from build123d import *

# Parameters (mm, degrees)
F0_W     = 200
F0_H     = 140
F1_DEPTH = 3
F2_R     = 10
F3_W     = 25
F3_H     = 50
F4_DEPTH = 20
F5_R     = 5
F6_DEPTH = 87.527208


with BuildPart() as f1:
    # F0 (on Front) → F1 (new body)
    with BuildSketch(Plane.XZ):
        with Locations((16.716758, -6.526925)):
            Rectangle(F0_W, F0_H)
    extrude(amount=F1_DEPTH)

    # F2
    f2_edges = [f1.edges().sort_by_distance(p)[0] for p in [
        (-83.283242, -1.5, -76.526925),
        (116.716758, -1.5, 63.473075),
        (116.716758, -1.5, -76.526925),
        (-83.283242, -1.5, 63.473075),
    ]]
    fillet(f2_edges, radius=F2_R)

    # F3 (on Front) → F4 (join)
    with BuildSketch(Plane.XZ):
        with Locations((129.216758, -6.526925)):
            Rectangle(F3_W, F3_H)
    extrude(amount=F4_DEPTH)

    # F5 (on face) → F6 (cut)
    with BuildSketch(Plane.XY.offset(18.473075)):
        with Locations((131.716758, -10)):
            Circle(F5_R)
    extrude(amount=-F6_DEPTH, mode=Mode.SUBTRACT)


solid = f1.part
Check sheet for the modelled part. Datum: model origin and axes. Units: mm. A direction names the side the tool comes from. Round coordinates to 2 decimals unless told otherwise and drop trailing zeros. Loops run counter-clockwise (first coordinate to the right, second up) from the corner with the lowest first, then second, coordinate; pieces in that order, holes last. Notation, with made-up numbers: M -28,25 L 9,25 A20 cw 9,45 Z; hole C -25,55 d7. An arc over 180 degrees is marked long. One line per item, written item: value.
(1) Depth check by flat-ended pin: pin 1 Ø2 at (x, z) = (112.5, 10) entering from -Y; pin 2 Ø5 at (y, z) = (-9, 4) entering from -X; pin 3 Ø0.9 at (y, z) = (-2, 27.5) entering from +X. Enter the tip coordinate at first touch or a pass-through.
Computed values:
pin 1: stops at y = -3
pin 2: stops at x = 116.72
pin 3: stops at x = 116.72
(2) Sectioned sample at D-D, the plane z = -64. Record the cut outline in (x, y), then the cut area to 3 significant figures.
Computed values:
outline: M -83.28,-3 L 116.72,-3 L 116.72,0 L -83.28,0 Z
area: 600 mm^2
(3) Sectioned sample at C-C, the plane x = 119. Record the cut outline in (y, z), then the cut area to 3 significant figures.
Computed values:
outline: M -20,-31.53 L 0,-31.53 L 0,18.47 L -20,18.47 Z
area: 1,000 mm^2
(4) Release check for a two-part mould opening along Y. For faces 1 (the face through (126, -10, -31.527)), 2 (the face through (28, 0, -6)), 3 (the face through (136.486, -8.498, -6.177)) record: +Y half, -Y half, draft (parallel to the pull), parting line (faces both ways), or undercut.
Computed values:
face 1: draft
face 2: +Y half
face 3: undercut
(5) Sectioned sample at B-B, the plane z = 6. Record the cut outline in (x, y).
Computed values:
outline: M -83.28,-3 L 116.72,-3 L 116.72,-20 L 141.72,-20 L 141.72,0 L -83.28,0 Z; hole C 131.72,-10 d10
(6) Access from +Z, -Z, +X, -X, +Y, -Y to the whole of each face (thin tool, end or side, straight path). Record for faces 4 (the face through (116.717, -11, -7)), 5 (the face through (126, -10, 18.473)), 6 (the face through (141.717, -10, -7)).
Computed values:
face 4: +Z, -Z, -X, -Y
face 5: +Z, +X, +Y, -Y
face 6: +Z, -Z, +X, +Y, -Y
(7) Thickness scan on line 1 (Y direction, x = 105, z = -31.5); line 2 (X direction, y = -2.25, z = -51); line 3 (Z direction, x = 129, y = -5.25). Record the ranges inside material, lowest first.
Computed values:
line 1: y = -3 to 0
line 2: x = -83.28 to 116.72
line 3: z = -31.53 to 18.47
(8) Sectioned sample at A-A, the plane y = -10. Record the cut outline in (x, z), then the cut area to 3 significant figures.
Computed values:
outline: M 116.72,-31.53 L 126.72,-31.53 L 126.72,18.47 L 116.72,18.47 Z; M 136.72,-31.53 L 141.72,-31.53 L 141.72,18.47 L 136.72,18.47 Z
area: 750 mm^2
